Source: CAD feature listing. Evaluate the final solid. Frame: model axes, mm. A direction names the side the tool comes from. Give positions to 0.01 mm unless a question says otherwise; leave off trailing zeros. Write each loop counter-clockwise with the first axis right and the second up, starting at its lowest first coordinate (ties: lowest second). Pieces come first, ordered by that corner, then holes. Notation, with made-up numbers: (20.5, 88.25) -> (73.5, 88.25) arc R18 ccw to (73.5, 113.25) -> close; hole circle Ø5 at (9, 29). An arc over 180 degrees is marked (long way). Use one line per item in the form item = value. Start each with the question number.
(1) Draft query along Y for faces 1 (the face through (9.93, 24.48, 10.14)), 2 (the face through (13.52, 1.05, 18.66)), 3 (the face through (3.57, -24.55, -9.52)). Return one class per face: pulls with the +Y half, pulls with the -Y half, needs draft (parallel to the pull), parting line crosses it, or undercut.
(2) Set-up query: faces 4 (the face through (3, -26, 0)), 5 (the face through (11.4, -20.6, -12.4)), 6 (the face through (0, -12, 0)). Return all of +Z, -Z, +X, -X, +Y, -Y with unobstructed straight access to the full face (end or side cutting, diameter ignored); none if empty.
(3) Cut plane B-B, the plane x = 6.25. Output: boundary loops of the cut face in (y, z).
(4) First-contact query: P1, Ø6, axis at x = 2.5, z = -2.5, coming from the -Y side; P2, Ø3, axis at x = 2, z = 20, coming from the -Y side; P3, Ø6, axis at y = 1, z = 16.5, coming from the -X side. Flat tips, straight axial feed; report the tip coordinate or a pass-through.
(5) Cut plane D-D, the plane y = 0. Count the separate pieces of the cut face and the enclosed holes in it, and give its area (3 significant figures).
(6) Material intervals for line 1 along Z through (x, y) = (8.75, 0); line 2 along Z through (x, y) = (11, -12); line 3 along Z through (x, y) = (9, -15), sorted ascending. Write a range as from..to.
(7) Cut plane C-C, the plane x = 13. Output: boundary loops of the cut face in (y, z), and give its area (3 significant figures).
(8) Cut plane A-A, the plane z = 0. Output: boundary loops of the cut face in (x, y), and give its area (3 significant figures).
from build123d import *

# Parameters (mm, degrees)
SKETCH1_R           = 32.5
BOSS_EXTRUDE1_DEPTH = 15
CUT_EXTRUDE1_START  = -12
SKETCH2_R           = 3.4999999999999996
CUT_EXTRUDE1_DEPTH  = 12
SKETCH2_3_R         = 3.4999999999999996
SKETCH2_3_R_2       = 3.5
SKETCH2_3_R_3       = 8
CUT_EXTRUDE2_DEPTH  = 49.34769901453429
CUT_EXTRUDE3_START  = -3
SKETCH2_4_R         = 3.5
SKETCH2_4_R_2       = 8
CUT_EXTRUDE3_DEPTH  = 12
FILLET1_R           = 2
FILLET2_R           = 2


with BuildPart() as part:
    # Sketch1 → Boss-Extrude1 (new body)
    with BuildSketch(Plane(origin=(0, 0, 0), x_dir=(0, 0, -1), z_dir=(1, 0, 0))):
        Circle(SKETCH1_R)
    extrude(amount=BOSS_EXTRUDE1_DEPTH)

    # Sketch2 → Cut-Extrude1 (cut)
    # profile 1 of 4: a face of its own
    with BuildSketch(Plane(origin=(15, 0, 0), x_dir=(0, 0, -1), z_dir=(1, 0, 0)).offset(CUT_EXTRUDE1_START)):
        with BuildLine():
            ThreePointArc((12.437211551865326, 30.026084806616858), (1.99e-15, 32.5), (-12.43721155186533, 30.026084806616854))
            Line((-12.437211551865326, 30.02608480661686), (-11.289161254770068, 27.254446209083))
            ThreePointArc((-11.289161254770706, 27.254446209082737), (-1.129e-14, 29.500000000000007), (11.28916125477069, 27.254446209082744))
            Line((11.289161254770068, 27.254446209083), (12.437211551865326, 30.02608480661686))
        make_face()
    # profile 2 of 4: a face of its own
    with BuildSketch(Plane(origin=(15, 0, 0), x_dir=(0, 0, -1), z_dir=(1, 0, 0)).offset(CUT_EXTRUDE1_START)):
        with BuildLine():
            ThreePointArc((11.28916125477069, 27.254446209082744), (-1.129e-14, 29.500000000000007), (-11.289161254770706, 27.254446209082737))
            Line((-11.289161254770068, 27.254446209083), (-7.778174593051978, 18.778174593052064))
            ThreePointArc((-7.778174593051979, 18.778174593052064), (4.4e-16, 13.580964487968082), (7.778174593051979, 18.778174593052064))
            Line((7.778174593051979, 18.778174593052064), (11.289161254770068, 27.254446209083))
        make_face()
        with Locations((0, 22)):
            Circle(SKETCH2_R, mode=Mode.SUBTRACT)
    # profile 3 of 4: a face of its own
    with BuildSketch(Plane(origin=(15, 0, 0), x_dir=(0, 0, -1), z_dir=(1, 0, 0)).offset(CUT_EXTRUDE1_START)):
        with BuildLine():
            Line((-7.778174593051979, -18.778174593052064), (-11.289161254770068, -27.254446209083))
            ThreePointArc((-11.2891612547707, -27.25444620908274), (-5.42e-15, -29.500000000000007), (11.28916125477069, -27.254446209082744))
            Line((11.289161254770068, -27.254446209083), (7.778174593051979, -18.778174593052064))
            ThreePointArc((7.778174593051979, -18.778174593052064), (4.4e-16, -13.580964487968082), (-7.778174593051979, -18.778174593052064))
        make_face()
        with Locations((-1.5363e-13, -22)):
            Circle(SKETCH2_R, mode=Mode.SUBTRACT)
    # profile 4 of 4: a face of its own
    with BuildSketch(Plane(origin=(15, 0, 0), x_dir=(0, 0, -1), z_dir=(1, 0, 0)).offset(CUT_EXTRUDE1_START)):
        with BuildLine():
            Line((-11.289161254770068, -27.254446209083), (-12.437211551865326, -30.02608480661686))
            ThreePointArc((-12.43721155186533, -30.026084806616854), (-5.97e-15, -32.5), (12.43721155186532, -30.02608480661686))
            Line((12.437211551865326, -30.02608480661686), (11.289161254770068, -27.254446209083))
            ThreePointArc((11.28916125477069, -27.254446209082744), (-5.42e-15, -29.500000000000007), (-11.2891612547707, -27.25444620908274))
        make_face()
    extrude(amount=CUT_EXTRUDE1_DEPTH, mode=Mode.SUBTRACT)

    # Sketch2<3> → Cut-Extrude2 (cut, through all)
    with BuildSketch(Plane(origin=(15, 0, 0), x_dir=(0, 0, -1), z_dir=(1, 0, 0))):
        with Locations((0, 22)):
            Circle(SKETCH2_3_R)
        with Locations((-1.5363e-13, -22)):
            Circle(SKETCH2_3_R)
        with Locations((-21.999999999999996, 2.3044e-13)):
            Circle(SKETCH2_3_R_2)
        with Locations((22, -7.681e-14)):
            Circle(SKETCH2_3_R_2)
        Circle(SKETCH2_3_R_3)
    extrude(amount=-CUT_EXTRUDE2_DEPTH, mode=Mode.SUBTRACT)

    # Sketch2<4> → Cut-Extrude3 (cut)
    with BuildSketch(Plane(origin=(15, 0, 0), x_dir=(0, 0, -1), z_dir=(1, 0, 0)).offset(CUT_EXTRUDE3_START)):
        with BuildLine():
            Line((-10.549813190585843, 17.630124295956804), (-14.002272700359098, 25.96509886799544))
            ThreePointArc((-14.002272700359109, 25.965098867995447), (-29.500000000000007, 3.61e-15), (-14.002272700359114, -25.965098867995444))
            Line((-14.0022727003591, -25.96509886799545), (-10.549813190585835, -17.630124295956804))
            ThreePointArc((-10.549813190585837, -17.630124295956804), (1.78e-15, -10.580964487968227), (10.549813190585844, -17.6301242959568))
            Line((10.549813190585843, -17.6301242959568), (14.0022727003591, -25.96509886799545))
            ThreePointArc((14.002272700359107, -25.965098867995447), (25.33097949804344, -15.119241967430227), (29.500000000000007, -7.23e-15))
            ThreePointArc((29.500000000000007, 0), (25.33097949804344, 15.119241967430227), (14.0022727003591, 25.96509886799545))
            Line((14.002272700359098, 25.96509886799544), (10.549813190585843, 17.630124295956804))
            ThreePointArc((10.549813190585843, 17.6301242959568), (-1.78e-15, 10.58096448796808), (-10.549813190585843, 17.630124295956804))
        make_face()
        with Locations((22, -7.681e-14)):
            Circle(SKETCH2_4_R, mode=Mode.SUBTRACT)
        with Locations((-21.999999999999996, 2.3044e-13)):
            Circle(SKETCH2_4_R, mode=Mode.SUBTRACT)
        Circle(SKETCH2_4_R_2, mode=Mode.SUBTRACT)
    extrude(amount=-CUT_EXTRUDE3_DEPTH, mode=Mode.SUBTRACT)

    # Fillet1
    fillet1_edges = [part.edges().sort_by_distance(p)[0] for p in [
        (6, -25.96509886799545, -14.002272700359104),
        (12, -10.580964487968227, -1.78e-15),
        (6, -25.965098867995447, 14.00227270035911),
        (6, 25.965098867995444, 14.002272700359104),
        (12, 21.79761158197612, 12.27604294547247),
        (12, 10.580964487968078, 3.11e-15),
        (12, 21.79761158197612, -12.27604294547247),
        (6, 25.965098867995444, -14.0022727003591),
        (12, 7.11e-15, 29.5),
        (12, -21.797611581976128, 12.276042945472469),
        (12, -21.797611581976128, -12.276042945472472),
        (12, -3.11e-15, -29.500000000000007),
    ]]
    fillet(fillet1_edges, radius=FILLET1_R)

    # Fillet2
    fillet2_edges = [part.edges().sort_by_distance(p)[0] for p in [
        (3, 24.40212969983446, 10.107693072458654),
        (3, 24.402129699834465, -10.107693072458654),
        (3, 13.580964487968082, -8.9e-16),
        (3, -24.40212969983446, 10.107693072458654),
        (3, -13.580964487968082, 8.9e-16),
        (3, -24.402129699834465, -10.107693072458652),
    ]]
    fillet(fillet2_edges, radius=FILLET2_R)


solid = part.part
Geometry says:
q1.face_1 = pulls with the +Y half
q1.face_2 = undercut
q1.face_3 = pulls with the -Y half
q2.face_4 = +X, -Y
q2.face_5 = -X
q2.face_6 = +Z, -Z, -X, +Y, -Y
q3.outline = (-30.03, -12.44) arc R32.5 ccw to (30.03, -12.44) -> (18.78, -7.78) arc R8.42 cw to (18.78, 7.78) -> (30.03, 12.44) arc R32.5 ccw to (-30.03, 12.44) -> (-18.78, 7.78) arc R8.42 cw to (-18.78, -7.78) -> close; hole (-24.75, -16.06) arc R29.5 ccw to (24.75, -16.06) arc R2 ccw to (23.84, -13.12) -> (17.63, -10.55) arc R11.42 cw to (17.63, 10.55) -> (23.84, 13.12) arc R2 ccw to (24.75, 16.06) arc R29.5 ccw to (-24.75, 16.06) arc R2 ccw to (-23.84, 13.12) -> (-17.63, 10.55) arc R11.42 cw to (-17.63, -10.55) -> (-23.84, -13.12) arc R2 ccw to start
q4.P1 = -32.5
q4.P2 = -26.72
q4.P3 = 12
q5.separate_pieces = 4
q5.enclosed_holes = 0
q5.area = 179 mm^2
q6.line_1 = -32.5..-29.5, 29.5..32.5
q6.line_2 = -30.2..-26.66, -6.05..6.05, 26.66..30.2
q6.line_3 = -28.83..-25.4, -9.02..-4.68, 4.68..9.02, 25.4..28.83
q7.outline = (-30.03, -12.44) arc R32.5 ccw to (30.03, -12.44) -> (18.78, -7.78) arc R8.42 cw to (18.78, 7.78) -> (30.03, 12.44) arc R32.5 ccw to (-30.03, 12.44) -> (-18.78, 7.78) arc R8.42 cw to (-18.78, -7.78) -> close; hole circle Ø16 at (0, 0); hole circle Ø7 at (0, -22); hole circle Ø7 at (0, 22)
q7.area = 2,390 mm^2
q8.outline = (0, -32.5) -> (3, -32.5) -> (3, -25.5) -> (0, -25.5) -> close; (0, -18.5) -> (3, -18.5) -> (3, -15.58) arc R2 cw to (5, -13.58) -> (15, -13.58) -> (15, -8) -> (12, -8) -> (12, -8.58) arc R2 cw to (10, -10.58) -> (0, -10.58) -> close; (0, 10.58) -> (10, 10.58) arc R2 cw to (12, 8.58) -> (12, 8) -> (15, 8) -> (15, 13.58) -> (5, 13.58) arc R2 cw to (3, 15.58) -> (3, 18.5) -> (0, 18.5) -> close; (0, 25.5) -> (3, 25.5) -> (3, 32.5) -> (0, 32.5) -> close
q8.area = 180 mm^2
